from build123d import *

# Parameters (mm, degrees)
SKETCH1_W           = 74.39914
SKETCH1_H           = 34.544
BOSS_EXTRUDE1_DEPTH = 5.08
SKETCH2_W           = 10.16
SKETCH2_H           = 6.35
BOSS_EXTRUDE2_DEPTH = 19.05
SKETCH3_R           = 0.635
CUT_EXTRUDE1_DEPTH  = 82.703658527
SKETCH4_W           = 19.05
SKETCH4_H           = 22.352
CUT_EXTRUDE2_DEPTH  = 85.210584066
SKETCH5_R           = 0.635
CUT_EXTRUDE3_DEPTH  = 86.503081048
SKETCH6_R           = 0.635
CUT_EXTRUDE4_DEPTH  = 81.098757273
CUT_EXTRUDE5_DEPTH  = 19.05


with BuildPart() as part:
    # Sketch1 → Boss-Extrude1 (new body)
    with BuildSketch(Plane(origin=(0, 0, 0), x_dir=(1, 0, 0), z_dir=(0, 1, 0))):
        with Locations((37.19957, 17.272)):
            Rectangle(SKETCH1_W, SKETCH1_H)
    extrude(amount=BOSS_EXTRUDE1_DEPTH)

    # Sketch2 → Boss-Extrude2 (add)
    with BuildSketch(Plane(origin=(0, 5.08, 0), x_dir=(1, 0, 0), z_dir=(0, 1, 0))):
        with Locations((69.31914, 20.447)):
            Rectangle(SKETCH2_W, SKETCH2_H)
        with Locations((5.08, 14.097)):
            Rectangle(SKETCH2_W, SKETCH2_H)
    extrude(amount=BOSS_EXTRUDE2_DEPTH)

    # Sketch3 → Cut-Extrude1 (cut, through all)
    with BuildSketch(Plane(origin=(0, 0, -23.622), x_dir=(-1, 0, 0), z_dir=(0, 0, -1))):
        with Locations((-69.31914, 20.828)):
            Circle(SKETCH3_R)
        with Locations((-69.31914, 14.732)):
            Circle(SKETCH3_R)
    extrude(amount=-CUT_EXTRUDE1_DEPTH, mode=Mode.SUBTRACT)

    # Sketch4 → Cut-Extrude2 (cut, through all)
    with BuildSketch(Plane(origin=(0, 5.08, 0), x_dir=(1, 0, 0), z_dir=(0, 1, 0))):
        with Locations((49.63414, 17.272)):
            Rectangle(SKETCH4_W, SKETCH4_H)
    extrude(amount=-CUT_EXTRUDE2_DEPTH, mode=Mode.SUBTRACT)

    # Sketch5 → Cut-Extrude3 (cut, through all)
    with BuildSketch(Plane(origin=(0, 0, 0), x_dir=(-1, 0, 0), z_dir=(0, -1, 0))):
        with Locations(Location((-5.08, 28.067, 0), (0, 0, 90))):
            Circle(SKETCH5_R)
        with Locations(Location((-30.48, 28.067, 0), (0, 0, 90))):
            Circle(SKETCH5_R)
        with Locations(Location((-30.48, 6.477, 0), (0, 0, 90))):
            Circle(SKETCH5_R)
        with Locations(Location((-5.08, 6.477, 0), (0, 0, 90))):
            Circle(SKETCH5_R)
    extrude(amount=-CUT_EXTRUDE3_DEPTH, mode=Mode.SUBTRACT)

    # Sketch6 → Cut-Extrude4 (cut, through all)
    with BuildSketch(Plane(origin=(0, 0, -17.272), x_dir=(-1, 0, 0), z_dir=(0, 0, -1))):
        with Locations((-5.08, 20.828)):
            Circle(SKETCH6_R)
        with Locations((-5.08, 14.732)):
            Circle(SKETCH6_R)
    extrude(amount=-CUT_EXTRUDE4_DEPTH, mode=Mode.SUBTRACT)

    # Sketch8 → Cut-Extrude5 (cut)
    with BuildSketch(Plane(origin=(0, 24.13, 0), x_dir=(1, 0, 0), z_dir=(0, 1, 0))):
        Polygon((10.16, 10.922), (8.255, 17.272), (10.16, 17.272), align=None)
    extrude(amount=-CUT_EXTRUDE5_DEPTH, mode=Mode.SUBTRACT)


solid = part.part
Can you work these out from the model? Positions are in its coordinate system, mm. A direction names the side the tool comes from. Give positions to 0.01 mm unless a question says otherwise; leave off trailing zeros. Order: outer loops, then holes, each group sorted by start corner. A loop starts at its lowest first (then second) coordinate and runs counter-clockwise, first axis right, second up. Notation, with made-up numbers: M -23.75,77.5 L 29.25,77.5 A10 cw 29.25,89.5 Z; hole C 53.25,27.25 d6. An arc over 180 degrees is marked long. Use one line per item in the form item = value. Start each with the question number.
Item 1: If we section it at A-A (y = 6.5): Write out the boundary of the cut face in (x, z) (3 decimals).
Item 2: If we section it at B-B (z = -14): Write out the boundary of the cut face in (x, y) (3 decimals).
Item 3: Will these pins go through, and if not, where does the flat tip stop? pin 1 Ø2 at (x, z) = (30.48, -6.477) entering from +Y; pin 2 Ø11 at (x, y) = (67, 13) entering from +Z; pin 3 Ø5 at (y, z) = (13, -22) entering from -X.
Item 4: If we section it at D-D (x = 58): Write out the boundary of the cut face in (y, z).
Item 5: If we section it at C-C (y = 3.5): Write out the boundary of the cut face in (x, z) (3 decimals).
Item 6: If I drill on line 1 along Y through (x, z) = (5.08, -13.5); line 2 along X through (y, z) = (5, -22.5); line 3 along Z through (x, y) = (8, 10.5), over which ranges is the centre line in solid material (lowest first)?
Item 7: For faces 5 (the flat face through (6, 14, -10.922)), 6 (the flat face through (64.239, 14, -20)), 7 (the flat face through (9.22, 14.74, -14.05)), 8 (the flat face through (68, 14, -23.622)), 9 (the flat face through (40.109, 3, -17)), which set-ups out of +Z, -Z, +X, -X, +Y, -Y let a thin tool reach every point of the face, with its end or its side?
Item 8: We'd pull the mould along X, two halves only. Please class faces 1 (the flat face through (50, 3, -28.448)), 2 (the flat face through (59.159, 3, -17)), 3 (the flat face through (0, 7, -17)), 4 (the flat face through (69, 24.13, -20)): +X half, -X half, draft (parallel to the pull), parting line (faces both ways), or undercut.
Outcome:
q1.outline = M 0,-17.272 L 8.255,-17.272 L 10.16,-10.922 L 0,-10.922 Z; M 64.239,-23.622 L 74.399,-23.622 L 74.399,-17.272 L 64.239,-17.272 Z
q2.outline = M 0,0 L 40.109,0 L 40.109,5.08 L 9.237,5.08 L 9.237,24.13 L 0,24.13 Z; M 59.159,0 L 74.399,0 L 74.399,5.08 L 59.159,5.08 Z; hole C 5.08,14.732 d1.27; hole C 5.08,20.828 d1.27
q3.pin_1 = 5.08
q3.pin_2 = -17.27
q3.pin_3 = 64.24
q4.outline = M 0,-34.54 L 5.08,-34.54 L 5.08,-28.45 L 0,-28.45 Z; M 0,-6.1 L 5.08,-6.1 L 5.08,0 L 0,0 Z
q5.outline = M 0,-34.544 L 74.399,-34.544 L 74.399,0 L 0,0 Z; hole C 5.08,-28.067 d1.27; hole C 5.08,-6.477 d1.27; hole C 30.48,-28.067 d1.27; hole C 30.48,-6.477 d1.27; hole M 40.109,-28.448 L 59.159,-28.448 L 59.159,-6.096 L 40.109,-6.096 Z
q6.line_1 = 0 to 14.1, 15.37 to 20.19, 21.46 to 24.13
q6.line_2 = 0 to 40.11, 59.16 to 74.4
q6.line_3 = -17.27 to -10.92
q7.face_5 = +Z, +X, -X, +Y
q7.face_6 = +Z, -Z, -X, +Y
q7.face_7 = -Z, +X, +Y
q7.face_8 = -Z, +X, -X, +Y
q7.face_9 = +Y, -Y
q8.face_1 = undercut
q8.face_2 = undercut
q8.face_3 = -X half
q8.face_4 = draft
